Build history of the part. All positions in model axes, mm. Coordinates: 2 decimals unless noted, no trailing zeros. Order: outer loops, then holes, each group sorted by start corner. A loop starts at its lowest first (then second) coordinate and runs counter-clockwise, first axis right, second up. Notation, with made-up numbers: M 63,26.5 L 94,26.5 A22 cw 94,55.5 Z; hole C 48.5,22.25 d6. An arc over 180 degrees is marked long. Write item = value, one per line. Start each with the question number.
Q1. Pull direction X, two halves, no side cores. Call faces 1 (the face through (64.484, -0.493, -110.236)), 2 (the face through (197, 0, -63)): released by +X, released by -X, zero draft, split by the parting line, or undercut.
Q2. Band-saw the part on A-A on y = -0.5. Write the cut outline in (x, z), plus the area to 3 significant figures.
Q3. Band-saw the part on B-B on z = -90. Write the cut outline in (x, y).
Q4. Drill centre lines: probe 1 along X at (y, z) = (-0.6, -50); probe 2 along X at (y, z) = (-0.3, -90); probe 3 along Z at (x, y) = (376, -0.5). Where is each one in solid material? Low to high.
```python
from build123d import *

# Parameters (mm, degrees)
SKETCH_2_W             = 400
SKETCH_2_H             = 125
SKETCH_2_R             = 2.5
SM_BASE_FLANGE_1_DEPTH = 1
SKETCH_3_R             = 25.5
CUT_EXTRUDE_1_DEPTH    = 420.077558454


# Sheet-metal steps are written as plain solids
with BuildPart() as part:
    # Sketch 2 → Базовая кромка1 (new body)
    with BuildSketch(Plane(origin=(0, 0, 0), x_dir=(1, 0, 0), z_dir=(0, 1, 0))):
        with Locations((200, 62.5)):
            Rectangle(SKETCH_2_W, SKETCH_2_H)
        with Locations(Location((24, 50, 0), (0, 0, 270))):
            Circle(SKETCH_2_R, mode=Mode.SUBTRACT)
        with Locations(Location((376, 50, 0), (0, 0, 90))):
            Circle(SKETCH_2_R, mode=Mode.SUBTRACT)
    extrude(amount=-SM_BASE_FLANGE_1_DEPTH)

    # Эскиз3 → Вырез-Вытянуть1 (cut, through all)
    with BuildSketch(Plane(origin=(0, 0, 0), x_dir=(1, 0, 0), z_dir=(0, 1, 0))):
        with Locations(Location((80, 90, 0), (0, 0, 270))):
            Circle(SKETCH_3_R)
    extrude(amount=-CUT_EXTRUDE_1_DEPTH, mode=Mode.SUBTRACT)


solid = part.part
```
Recorded:
q1.face_1 = undercut
q1.face_2 = zero draft
q2.outline = M 0,-125 L 400,-125 L 400,0 L 0,0 Z; hole C 24,-50 d5; hole C 80,-90 d51; hole C 376,-50 d5
q2.area = 47,900 mm2
q3.outline = M 0,-1 L 54.5,-1 L 54.5,0 L 0,0 Z; M 105.5,-1 L 400,-1 L 400,0 L 105.5,0 Z
q4.probe_1 = 0 to 21.5, 26.5 to 373.5, 378.5 to 400
q4.probe_2 = 0 to 54.5, 105.5 to 400
q4.probe_3 = -125 to -52.5, -47.5 to 0
